Design review of the part built by this model. Coordinates are the model's own, in mm. A direction names the side the tool comes from. Coordinates: 2 decimals unless noted, no trailing zeros. Write each loop counter-clockwise with the first axis right and the second up, starting at its lowest first coordinate (ties: lowest second). Pieces come first, ordered by that corner, then holes. Notation, with made-up numbers: M 35.5,34.5 L 72.5,34.5 A9 ccw 72.5,49.5 Z; hole C 81,40.5 d8. An arc over 180 degrees is marked long. Return JSON: item names as keys, results as strings. Group by question number.
```python
from build123d import *

# Parameters (mm, degrees)
SKETCH_R      = 4.2
PAD_DEPTH     = 2
SKETCH001_R   = 7.5
SKETCH001_R_2 = 4.6
PAD001_DEPTH  = 0.5
CHAMFER_SIZE  = 0.2


with BuildPart() as part:
    # Sketch → Pad (new body)
    with BuildSketch(Plane.XY):
        Polygon((6.350853, 0), (3.175426, 5.5), (-3.175426, 5.5), (-6.350853, 0), (-3.175426, -5.5), (3.175426, -5.5), align=None)
        Circle(SKETCH_R, mode=Mode.SUBTRACT)
    extrude(amount=PAD_DEPTH)

    # Sketch001 → Pad001 (join)
    with BuildSketch(Plane.XY):
        Circle(SKETCH001_R)
        Circle(SKETCH001_R_2, mode=Mode.SUBTRACT)
    extrude(amount=-PAD001_DEPTH)

    # Chamfer
    chamfer_edges = [part.edges().sort_by_distance(p)[0] for p in [
        (-4.2, 0, 2),
        (-4.76314, 2.75, 2),
        (-4.76314, -2.75, 2),
        (0, -5.5, 2),
        (4.76314, -2.75, 2),
        (4.76314, 2.75, 2),
        (0, 5.5, 2),
    ]]
    chamfer(chamfer_edges, length=CHAMFER_SIZE)


solid = part.part
```
Item 1: For pin 1 (3 mm diameter, centred on x = -5.5, y = 2, fed in from +Z); pin 2 (0.5 mm diameter, centred on x = 1, z = 1, fed in from +Y); pin 3 (1 mm diameter, centred on x = -4, z = 0, fed in from -Y); pin 4 (1.4 mm diameter, centred on x = -1.5, z = 0.5, fed in from -Y), all flat-tipped, find the tip position at first contact; note any pin that passes through.
Item 2: Machinability: for faces 1 (the flat face through (0, 5.5, 1)), 2 (the flat face through (0, -6, 0)), 3 (the cylindrical face through (-3.65, -2.8, -0.25)), 4 (the flat face through (4.74, -2.79, 0.89)), which of the approach directions +Z, -Z, +X, -X, +Y, -Y give a long, thin tool a straight path to every point of the face, cutting with its end or side? Answer none if there is none.
Item 3: Add section B-B (z = 0.3). Write out the cut boundary in (x, y), plus the area to 3 significant figures.
Item 4: Add section A-A (x = 0). Write out the cut boundary in (y, z), plus the area to 3 significant figures.
Item 5: For line 1 (Y direction, x = 0, z = 0.55); line 2 (Y direction, x = 0, z = -0.2); line 3 (Z direction, x = 6.25, y = -3.25), list the stretches that pass through material, from the lowest coordinate up.
Item 6: The part is to be moulded in two halves that separate along X. For faces 5 (the cylindrical face through (4.006, 1.262, 0.887)), 6 (the flat face through (3, 4, 2)), 7 (the flat face through (-4.74, 2.79, 0.89)), say which applies: pulls with the +X half, pulls with the -X half, needs draft (parallel to the pull), parting line crosses it, or undercut.
Geometry check:
{
 "1": {"pin 1": "z = 2", "pin 2": "y = 5.5", "pin 3": "y = -6.63", "pin 4": "y = -7.43"},
 "2": {"face 1": "+Z, +X, -X, +Y", "face 2": "+Z", "face 3": "-Z", "face 4": "+Z, +X, -Y"},
 "3": {"outline": "M -6.35,0 L -3.18,-5.5 L 3.18,-5.5 L 6.35,0 L 3.18,5.5 L -3.18,5.5 Z; hole C 0,0 d8.4", "area": "49.4 mm^2"},
 "4": {"outline": "M -7.5,-0.5 L -4.6,-0.5 L -4.6,0 L -4.2,0 L -4.2,1.8 L -4.4,2 L -5.3,2 L -5.5,1.8 L -5.5,0 L -7.5,0 Z; M 4.2,0 L 4.6,0 L 4.6,-0.5 L 7.5,-0.5 L 7.5,0 L 5.5,0 L 5.5,1.8 L 5.3,2 L 4.4,2 L 4.2,1.8 Z", "area": "8.02 mm^2"},
 "5": {"line 1": "-5.5 to -4.2, 4.2 to 5.5", "line 2": "-7.5 to -4.6, 4.6 to 7.5", "line 3": "-0.5 to 0"},
 "6": {"face 5": "undercut", "face 6": "needs draft", "face 7": "pulls with the -X half"}
}
